```python
from build123d import *

# Parameters (mm, degrees)
ESQUISSE1_R        = 1.5
ESQUISSE1_R_2      = 7.5
ESQUISSE1_R_3      = 1.6
BOSS_EXTRU_1_DEPTH = 4


with BuildPart() as part:
    # Esquisse1 → Boss.-Extru.1 (new body)
    with BuildSketch(Plane.XY):
        Polygon((-443.856361675, 119.15022686), (-49.513215925, 119.15022686), (-67.190885454, 101.472557331), (-64.36245833, 98.644130206), (-46.6847888, 116.321799736), (-46.6847888, -178.021346015), (-64.36245833, -160.343676485), (-67.190885454, -163.17210361), (-49.513215925, -180.84977314), (-443.856361675, -180.84977314), (-426.178692146, -163.17210361), (-429.00711927, -160.343676485), (-446.6847888, -178.021346015), (-446.6847888, 116.321799736), (-429.00711927, 98.644130206), (-426.178692146, 101.472557331), align=None)
        with Locations((-236.6397888, 25.29522686)):
            Circle(ESQUISSE1_R, mode=Mode.SUBTRACT)
        with Locations((-93.1297888, 25.29522686)):
            Circle(ESQUISSE1_R, mode=Mode.SUBTRACT)
        with Locations((-236.6397888, -59.79477314)):
            Circle(ESQUISSE1_R, mode=Mode.SUBTRACT)
        with Locations((-93.1297888, -59.79477314)):
            Circle(ESQUISSE1_R, mode=Mode.SUBTRACT)
        with Locations((-104.5597888, -133.60477314)):
            Circle(ESQUISSE1_R_2, mode=Mode.SUBTRACT)
        with Locations((-347.5347888, -49.04977314)):
            Circle(ESQUISSE1_R_3, mode=Mode.SUBTRACT)
        with Locations((-319.6347888, -49.04977314)):
            Circle(ESQUISSE1_R_3, mode=Mode.SUBTRACT)
        with Locations((-352.6347888, 3.05022686)):
            Circle(ESQUISSE1_R_3, mode=Mode.SUBTRACT)
        with Locations((-304.4347888, 1.75022686)):
            Circle(ESQUISSE1_R_3, mode=Mode.SUBTRACT)
        with Locations((-145.1997888, -133.60477314)):
            Circle(ESQUISSE1_R_2, mode=Mode.SUBTRACT)
        with Locations((-182.0297888, -133.60477314)):
            Circle(ESQUISSE1_R_2, mode=Mode.SUBTRACT)
        with Locations((-222.6697888, -133.60477314)):
            Circle(ESQUISSE1_R_2, mode=Mode.SUBTRACT)
    extrude(amount=BOSS_EXTRU_1_DEPTH)


solid = part.part
```
Work out the finished part from the listing and answer in its coordinate system (mm). A direction names the side the tool comes from. Coordinates: 2 decimals unless noted, no trailing zeros. Loops run counter-clockwise (first coordinate to the right, second up) from the corner with the lowest first, then second, coordinate; pieces in that order, holes last.
1) Consider probe 1 along X at (y, z) = (3.5, 1.65); probe 2 along Y at (x, z) = (-428.5, 0.5); probe 3 along X at (y, z) = (-140.5, 3.35). Determine where each line is inside the solid, lowest interval first.
Results:
probe 1: x = -446.68 to -354.17, -351.1 to -46.68
probe 2: y = -180.85 to -165.49, -160.85 to 99.15, 103.79 to 119.15
probe 3: x = -446.68 to -225.62, -219.72 to -184.98, -179.08 to -148.15, -142.25 to -107.51, -101.61 to -46.68
2) For faces 1 (the flat face through (-244, -29, 0)), 2 (the flat face through (-434.894, 110.188, 1.972)), determine the directions among +Z, -Z, +X, -X, +Y, -Y from which every point of the face is accessible in a straight line to the end or side of a thin tool.
Results:
face 1: -Z, +X, -X, +Y, -Y
face 2: +Z, -Z
3) For a pull along X with two mould halves and no side action, classify faces 3 (the cylindrical face through (-150.73, -128.54, 1.97)), 4 (the flat face through (-437.97, 107.607, 1.972)), 5 (the flat face through (-244, -29, 4)) as +X half, -X half, draft (parallel to the pull), parting line (faces both ways), or undercut.
Results:
face 3: undercut
face 4: undercut
face 5: draft
4) A flat-ended cylindrical pin translates along its axis: pin 1 (2 mm diameter, centred on x = -251.5, y = -19.5, fed in from -Z). Find the tip coordinate at first contact, or state that the pin passes through.
Results:
pin 1: stops at z = 0
5) Section A-A (x = -223) is taken. Give the vertices of the cut face in (y, z), plus the area to 3 significant figures.
Results:
outline: (-180.85, 0) - (-141.1, 0) - (-141.1, 4) - (-180.85, 4) - close; (-126.11, 0) - (119.15, 0) - (119.15, 4) - (-126.11, 4) - close
area: 1,140 mm2
